```python
from build123d import *

# Parameters (mm, degrees)
F0_W      = 4.1
F0_H      = 2.55
F0_W_2    = 3.1
F0_H_2    = 1.55
F2_DEPTH  = 168.1
F0_R      = 9.525
F3_DEPTH  = 6.35
F6_W      = 4.1
F6_H      = 2.55
F6_W_2    = 3.1
F6_H_2    = 1.55
F7_DEPTH  = 28.7
F8_R      = 9.525
F8_W      = 4.1
F8_H      = 2.55
F9_DEPTH  = 6.35
F4_R      = 9.525
F4_W      = 4.1
F4_H      = 2.55
F10_DEPTH = 6.35


with BuildPart() as f2:
    # F0 (on Front) → F2 (new body)
    with BuildSketch(Plane.XZ):
        Rectangle(F0_W, F0_H)
        Rectangle(F0_W_2, F0_H_2, mode=Mode.SUBTRACT)
    extrude(amount=F2_DEPTH)

    # F0 (on Front) → F3 (join)
    with BuildSketch(Plane.XZ):
        Circle(F0_R)
        Rectangle(F0_W, F0_H, mode=Mode.SUBTRACT)
    extrude(amount=F3_DEPTH)

    # F6 (on offset) → F7 (join)
    with BuildSketch(Plane.XY.offset(1.275)):
        with Locations((0, -22.4)):
            Rectangle(F6_W, F6_H)
        with Locations((0, -22.4)):
            Rectangle(F6_W_2, F6_H_2, mode=Mode.SUBTRACT)
    extrude(amount=F7_DEPTH)

    # F8 (on face) → F9 (join)
    with BuildSketch(Plane.XY.offset(29.975)):
        with Locations((0, -22.4)):
            Circle(F8_R)
        with Locations((0, -22.4)):
            Rectangle(F8_W, F8_H, mode=Mode.SUBTRACT)
    extrude(amount=-F9_DEPTH)

    # F4 (on face) → F10 (join)
    with BuildSketch(Plane.XZ.offset(168.1)):
        Circle(F4_R)
        Rectangle(F4_W, F4_H, mode=Mode.SUBTRACT)
    extrude(amount=-F10_DEPTH)


solid = f2.part
```
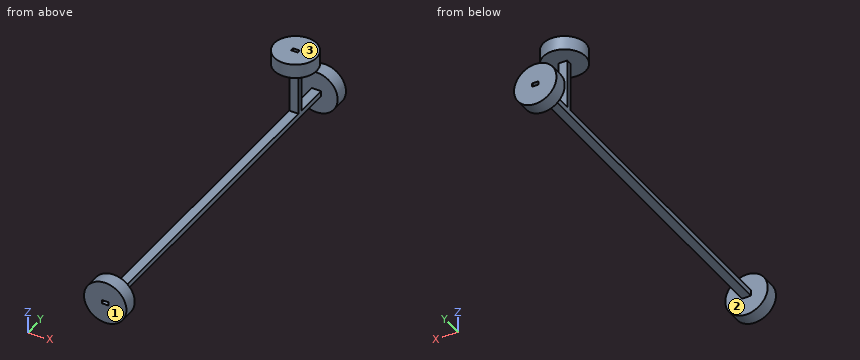
Build history of the part. All positions in model axes, mm. Face numbers are marked on the shaded views. Round coordinates to 2 decimals unless told otherwise and drop trailing zeros. Write each loop counter-clockwise with the first axis right and the second up, starting at its lowest first coordinate (ties: lowest second). Pieces come first, ordered by that corner, then holes.
1) Band-saw the part on D-D, the plane z = 20. List the corners of the cut face in (x, y) (3 decimals).
2) Band-saw the part on A-A, the plane y = -18.5. List the corners of the cut face in (x, z) (3 decimals), and give its area (3 significant figures).
3) Band-saw the part on C-C, the plane y = -57. List the corners of the cut face in (x, z) (3 decimals).
4) Mould opens along Y. For the marked faces 1, 2 and 3 say: +Y half, -Y half, draft (parallel to the pull), parting line (faces both ways), or undercut.
5) Band-saw the part on B-B, the plane x = 0. List the corners of the cut face in (y, z) (3 decimals).
6) Pin check, flat tips, straight feed: pin 1 (1.6 mm diameter, centred on x = 0.5, z = 13.5, fed in from -Y) (3 decimals); pin 2 (0.8 mm diameter, centred on y = -22.5, z = 14.5, fed in from +X); pin 3 (2 mm diameter, centred on x = -0.5, y = -59, fed in from +Z) (3 decimals). Stop position of each tip, or through.
7) Drill centre lines: probe 1 along Y at (x, z) = (1.75, 7) (3 decimals); probe 2 along Y at (x, z) = (5.75, -0.5); probe 3 along Z at (x, y) = (-1.75, -30) (3 decimals). Where is each one in solid material? Low to high.
Ans:
1. outline: (-2.05, -23.675) - (2.05, -23.675) - (2.05, -21.125) - (-2.05, -21.125) - close; hole (-1.55, -23.175) - (1.55, -23.175) - (1.55, -21.625) - (-1.55, -21.625) - close
2. outline: (-8.69, 23.625) - (8.69, 23.625) - (8.69, 29.975) - (-8.69, 29.975) - close; (-2.05, -1.275) - (2.05, -1.275) - (2.05, 1.275) - (-2.05, 1.275) - close; hole (-1.55, -0.775) - (1.55, -0.775) - (1.55, 0.775) - (-1.55, 0.775) - close
2. area: 116 mm2
3. outline: (-2.05, -1.275) - (2.05, -1.275) - (2.05, 1.275) - (-2.05, 1.275) - close; hole (-1.55, -0.775) - (1.55, -0.775) - (1.55, 0.775) - (-1.55, 0.775) - close
4. face 1: -Y half
4. face 2: undercut
4. face 3: draft
5. outline: (-168.1, -9.525) - (-161.75, -9.525) - (-161.75, -1.275) - (-6.35, -1.275) - (-6.35, -9.525) - (0, -9.525) - (0, -0.775) - (-168.1, -0.775) - close; (-168.1, 0.775) - (0, 0.775) - (0, 9.525) - (-6.35, 9.525) - (-6.35, 1.275) - (-21.125, 1.275) - (-21.125, 23.625) - (-12.875, 23.625) - (-12.875, 29.975) - (-21.625, 29.975) - (-21.625, 1.275) - (-23.175, 1.275) - (-23.175, 29.975) - (-31.925, 29.975) - (-31.925, 23.625) - (-23.675, 23.625) - (-23.675, 1.275) - (-161.75, 1.275) - (-161.75, 9.525) - (-168.1, 9.525) - close
6. pin 1: stops at y = -23.675
6. pin 2: stops at x = 2.05
6. pin 3: stops at z = 1.275
7. probe 1: y = -168.1 to -161.75, -23.675 to -21.125, -6.35 to 0
7. probe 2: y = -168.1 to -161.75, -6.35 to 0
7. probe 3: z = -1.275 to 1.275, 23.625 to 29.975
